Autodesk Inventor part; units mm, degrees
ref_plane "YZ Plane" through (0, 0, 0) normal (1, 0, 0) x (0, 1, 0)
ref_plane "XZ Plane" through (0, 0, 0) normal (0, 1, 0) x (-1, 0, 0)
ref_plane "XY Plane" through (0, 0, 0) normal (0, 0, 1) x (1, 0, 0)
sketch "Sketch1" plane through (0, 0, 0) normal (0, 0, 1) x (1, 0, 0)
  circle A0 centre (0, 0) radius 152.4
  circle A1 centre (0, 0) radius 6.35
  dimension "d0" = 304.8
  dimension "d1" = 12.7
extrude "Extrusion1" add sketch "Sketch1" along normal blind 50.8
sketch "Sketch2" plane through (0, 0, 50.8) normal (0, 0, 1) x (1, 0, 0)
  circle A0 centre (0, 0) radius 6.35
  circle A1 centre (0, 0) radius 38.1 construction
  circle A2 centre (0, 0) radius 101.6 construction
  line L0 (7.5, -37.3545) -> (15.7954, -100.3647)
  line L1 (-7.5, -37.3545) -> (-15.7954, -100.3647)
  line L2 (7.5, -37.3545) -> (-7.5, -37.3545) construction
  arc A3 (-15.7954, -100.3647) -> (15.7954, -100.3647) centre (0, 0) ccw
  arc A4 (-7.5, -37.3545) -> (7.5, -37.3545) centre (0, 0) ccw
  circle A5 centre (0, 0) radius 38.1 construction
  circle A6 centre (0, 0) radius 101.6 construction
  line L3 (36.1, -12.1821) -> (94.8161, -36.5031)
  line L4 (28.6, -25.1724) -> (79.0206, -63.8616)
  line L5 (36.1, -12.1821) -> (28.6, -25.1724) construction
  arc A7 (79.0206, -63.8616) -> (94.8161, -36.5031) centre (0, 0) ccw
  arc A8 (28.6, -25.1724) -> (36.1, -12.1821) centre (0, 0) ccw
  circle A9 centre (0, 0) radius 38.1 construction
  circle A10 centre (0, 0) radius 101.6 construction
  line L6 (28.6, 25.1724) -> (79.0206, 63.8616)
  line L7 (36.1, 12.1821) -> (94.8161, 36.5031)
  line L8 (28.6, 25.1724) -> (36.1, 12.1821) construction
  arc A11 (94.8161, 36.5031) -> (79.0206, 63.8616) centre (0, 0) ccw
  arc A12 (36.1, 12.1821) -> (28.6, 25.1724) centre (0, 0) ccw
  circle A13 centre (0, 0) radius 38.1 construction
  circle A14 centre (0, 0) radius 101.6 construction
  line L9 (-7.5, 37.3545) -> (-15.7954, 100.3647)
  line L10 (7.5, 37.3545) -> (15.7954, 100.3647)
  line L11 (-7.5, 37.3545) -> (7.5, 37.3545) construction
  arc A15 (15.7954, 100.3647) -> (-15.7954, 100.3647) centre (0, 0) ccw
  arc A16 (7.5, 37.3545) -> (-7.5, 37.3545) centre (0, 0) ccw
  circle A17 centre (0, 0) radius 38.1 construction
  circle A18 centre (0, 0) radius 101.6 construction
  line L12 (-36.1, 12.1821) -> (-94.8161, 36.5031)
  line L13 (-28.6, 25.1724) -> (-79.0206, 63.8616)
  line L14 (-36.1, 12.1821) -> (-28.6, 25.1724) construction
  arc A19 (-79.0206, 63.8616) -> (-94.8161, 36.5031) centre (0, 0) ccw
  arc A20 (-28.6, 25.1724) -> (-36.1, 12.1821) centre (0, 0) ccw
  circle A21 centre (0, 0) radius 38.1 construction
  circle A22 centre (0, 0) radius 101.6 construction
  line L15 (-28.6, -25.1724) -> (-79.0206, -63.8616)
  line L16 (-36.1, -12.1821) -> (-94.8161, -36.5031)
  line L17 (-28.6, -25.1724) -> (-36.1, -12.1821) construction
  arc A23 (-94.8161, -36.5031) -> (-79.0206, -63.8616) centre (0, 0) ccw
  arc A24 (-36.1, -12.1821) -> (-28.6, -25.1724) centre (0, 0) ccw
  point P0 (0, -37.3545)
  point P1 (0, -101.6)
  point P2 (32.35, -18.6773)
  point P3 (87.9882, -50.8)
  point P4 (32.35, 18.6773)
  point P5 (87.9882, 50.8)
  point P6 (0, 37.3545)
  point P7 (0, 101.6)
  point P8 (-32.35, 18.6773)
  point P9 (-87.9882, 50.8)
  point P10 (-32.35, -18.6773)
  point P11 (-87.9882, -50.8)
  dimension "d4" = 15
  dimension "d5" = 15
  dimension "d6" = 76.2
  dimension "d7" = 203.2
  dimension "d10" = 360
extrude "Extrusion2" cut sketch "Sketch2" against normal through all
sketch "Sketch3" plane through (0, 0, 50.8) normal (0, 0, 1) x (1, 0, 0)
  circle A0 centre (0, 0) radius 114.3
  dimension "d14" = 228.6
extrude "Extrusion3" cut sketch "Sketch3" against normal blind 10
sketch "Sketch4" plane through (0, 0, 0) normal (0, 0, -1) x (-1, 0, 0)
  circle A0 centre (0, 0) radius 6.35
  circle A1 centre (0, 0) radius 114.3
extrude "Extrusion4" cut sketch "Sketch4" against normal blind 10 contours A0 | A1
fillet "Fillet1" radius 12.7 2 edges at (-152.4, 0, 0) (-152.4, 0, 50.8)
properties part number "12 in Wheel"
The listing builds one solid part. Answer for the finished solid, in the listing's coordinates (mm). A direction names the side the tool comes from. Coordinates: 2 decimals unless noted, no trailing zeros. Loops run counter-clockwise (first coordinate to the right, second up) from the corner with the lowest first, then second, coordinate; pieces in that order, holes last. Notation, with made-up numbers: (55, -11) -> (103, -11) arc R37 ccw to (103, 25) -> close; hole circle Ø11 at (69.5, 58.5). An arc over 180 degrees is marked (long way). Return JSON: item names as keys, results as strings. Group by question number.
(1) A cutting plane is placed at D-D on x = 86. Count the separate pieces of the cut face and the enclosed holes in it, and give its area (3 significant figures).
(2) A cutting plane is placed at C-C on z = 29. Write down the section's boundary in (x, y), and give its area (3 significant figures).
(3) Determine the mould class of faces 1 (the cylindrical face through (-120.94, 92.73, 25.22)), 2 (the flat face through (-114.5, 0.7, 50.8)), 3 (the cylindrical face through (-114.19, 5.03, 45.87)) for opening direction X: released by +X, released by -X, zero draft, split by the parting line, or undercut.
(4) A cutting plane is placed at A-A on x = 0. Write down the section's boundary in (y, z).
(5) Find the intervals of material crossed by probe 1 along Y at (x, z) = (76, 38.5); probe 2 along Y at (x, z) = (-2.5, 26); probe 3 along Y at (x, z) = (-63.5, 16), in increasing order. Write a range as from..to.
(6) A cutting plane is placed at B-B on y = 0. Write down the section's boundary in (x, z), and give its area (3 significant figures).
(7) Which of the six approach directions +Z, -Z, +X, -X, +Y, -Y give full straight-line access (tool end or side, diameter ignored) to faces 4 (the flat face through (-24, 2, 10)), 5 (the flat face through (24, 2, 40.8)), 6 (the flat face through (53.46, 44.25, 25.62))?
(8) Given pin 1 Ø5 at (x, y) = (-40, -104) entering from -Z; pin 2 Ø1.5 at (y, z) = (-27.5, 6.5) entering from +X; pin 3 Ø5 at (x, z) = (-13, 19) entering from -Y, each flat-ended and moving along its own axis, determine where each tip first touches the part or whether it passes through.
The answers:
{
 "1": {"separate pieces": "3", "enclosed holes": "0", "area": "8,290 mm^2"},
 "2": {"outline": "circle Ø304.8 at (0, 0); hole (-94.82, -36.5) arc R101.6 ccw to (-79.02, -63.86) -> (-28.6, -25.17) arc R38.1 cw to (-36.1, -12.18) -> close; hole (-94.82, 36.5) -> (-36.1, 12.18) arc R38.1 cw to (-28.6, 25.17) -> (-79.02, 63.86) arc R101.6 ccw to start; hole (-15.8, -100.36) arc R101.6 ccw to (15.8, -100.36) -> (7.5, -37.35) arc R38.1 cw to (-7.5, -37.35) -> close; hole (-15.8, 100.36) -> (-7.5, 37.35) arc R38.1 cw to (7.5, 37.35) -> (15.8, 100.36) arc R101.6 ccw to start; hole circle Ø12.7 at (0, 0); hole (28.6, -25.17) -> (79.02, -63.86) arc R101.6 ccw to (94.82, -36.5) -> (36.1, -12.18) arc R38.1 cw to start; hole (28.6, 25.17) arc R38.1 cw to (36.1, 12.18) -> (94.82, 36.5) arc R101.6 ccw to (79.02, 63.86) -> close", "area": "63,900 mm^2"},
 "3": {"face 1": "split by the parting line", "face 2": "zero draft", "face 3": "undercut"},
 "4": {"outline": "(-152.4, 12.7) arc R12.7 ccw to (-139.7, 0) -> (-114.3, 0) -> (-114.3, 10) -> (-101.6, 10) -> (-101.6, 40.8) -> (-114.3, 40.8) -> (-114.3, 50.8) -> (-139.7, 50.8) arc R12.7 ccw to (-152.4, 38.1) -> close; (-38.1, 10) -> (-6.35, 10) -> (-6.35, 40.8) -> (-38.1, 40.8) -> close; (6.35, 10) -> (38.1, 10) -> (38.1, 40.8) -> (6.35, 40.8) -> close; (101.6, 10) -> (114.3, 10) -> (114.3, 0) -> (139.7, 0) arc R12.7 ccw to (152.4, 12.7) -> (152.4, 38.1) arc R12.7 ccw to (139.7, 50.8) -> (114.3, 50.8) -> (114.3, 40.8) -> (101.6, 40.8) -> close"},
 "5": {"probe 1": "y = -132.09..-61.54, -28.71..28.71, 61.54..132.09", "probe 2": "y = -152.38..-101.57, -38.02..-5.84, 5.84..38.02, 101.57..152.38", "probe 3": "y = -138.54..-51.95, -23.53..23.53, 51.95..138.54"},
 "6": {"outline": "(-152.4, 12.7) arc R12.7 ccw to (-139.7, 0) -> (-114.3, 0) -> (-114.3, 10) -> (-6.35, 10) -> (-6.35, 40.8) -> (-114.3, 40.8) -> (-114.3, 50.8) -> (-139.7, 50.8) arc R12.7 ccw to (-152.4, 38.1) -> close; (6.35, 10) -> (114.3, 10) -> (114.3, 0) -> (139.7, 0) arc R12.7 ccw to (152.4, 12.7) -> (152.4, 38.1) arc R12.7 ccw to (139.7, 50.8) -> (114.3, 50.8) -> (114.3, 40.8) -> (6.35, 40.8) -> close", "area": "10,400 mm^2"},
 "7": {"face 4": "-Z", "face 5": "+Z", "face 6": "+Z, -Z"},
 "8": {"pin 1": "stops at z = 10", "pin 2": "stops at x = 148.67", "pin 3": "stops at y = -152.04"}
}
